Geometry: final body of the model. Coordinates: model frame, mm. A direction names the side the tool comes from. Coordinates: 2 decimals unless noted, no trailing zeros. Write each loop counter-clockwise with the first axis right and the second up, starting at its lowest first coordinate (ties: lowest second). Pieces come first, ordered by that corner, then holes. Notation, with made-up numbers: (69, -27) -> (91, -27) arc R21 ccw to (91, 12) -> close; hole circle Ø11 at (76.25, -1.5). An arc over 180 degrees is marked (long way). One line per item, written item: value.
Autodesk Inventor part; units mm, degrees
ref_plane "YZ Plane" through (0, 0, 0) normal (1, 0, 0) x (0, 1, 0)
ref_plane "XZ Plane" through (0, 0, 0) normal (0, 1, 0) x (-1, 0, 0)
ref_plane "XY Plane" through (0, 0, 0) normal (0, 0, 1) x (1, 0, 0)
sketch "Sketch1" plane through (0, 0, 0) normal (0, 0, 1) x (1, 0, 0)
  line L0 (35, -3.75) -> (-35, -3.75)
  line L1 (-35, -3.75) -> (-35, 3.75)
  line L2 (-35, 3.75) -> (35, 3.75)
  line L3 (35, 3.75) -> (35, -3.75)
  line L4 (35, -3.75) -> (-35, 3.75) construction
  line L5 (-35, -3.75) -> (35, 3.75) construction
  line L6 (21.5, -16.5) -> (-21.5, -16.5)
  line L7 (-21.5, -16.5) -> (-21.5, 16.5)
  line L8 (-21.5, 16.5) -> (21.5, 16.5)
  line L9 (21.5, 16.5) -> (21.5, -16.5)
  line L10 (21.5, -16.5) -> (-21.5, 16.5) construction
  line L11 (-21.5, -16.5) -> (21.5, 16.5) construction
  line L12 (-35, -3.75) -> (-21.5, -16.5)
  line L13 (-35, 3.75) -> (-21.5, 16.5)
  arc A0 (32.3113, 4.5234) -> (35, 3.75) centre (34.605, 7.4371) ccw
  line L14 (21.5, -16.5) -> (35, -3.75)
  line L15 (35, 3.75) -> (21.5, 16.5)
  point P0 (0, 0)
  dimension "d0" = 70
  dimension "d1" = 7.5
  dimension "d2" = 43
  dimension "d3" = 33
extrude "Extrusion1" add sketch "Sketch1" along normal blind 30
sketch "Sketch2" plane through (-21.5, -16.5, 0) normal (0, -1, 0) x (1, 0, 0)
  line L0 (43, 30) -> (0, 30)
  line L1 (43, 0) -> (0, 0)
  line L2 (0, 30) -> (43, 30)
  line L3 (43, 30) -> (43, 0)
  line L4 (43, 0) -> (0, 0)
  line L5 (0, 0) -> (0, 30)
  line L6 (21.5, 30) -> (24.75, 30)
  line L7 (56.5, 0) -> (56.5, 30)
  line L8 (56.5, 0) -> (56.5, 10)
  line L9 (24.75, 30) -> (29.6997, 25.0503)
  arc A0 (29.6997, 25.0503) -> (56.5, 10) centre (56.5, 41.387) ccw
  arc A1 (55.355, 10.0209) -> (56.5, 10) centre (56.5, 41.387) ccw
  line L10 (56.5, 10) -> (46.9475, 10)
  line L11 (21.5, 30) -> (21.5, 26.75)
  line L12 (21.5, 30) -> (18.25, 30)
  line L13 (-13.5, 0) -> (-13.5, 30)
  line L14 (18.25, 30) -> (13.3003, 25.0503)
  arc A2 (-13.5, 10) -> (13.3003, 25.0503) centre (-13.5, 41.387) ccw
  line L15 (43, 30) -> (56.5, 30)
  line L16 (43, 0) -> (43, 30)
  line L17 (56.5, 30) -> (43, 30)
  line L18 (43, 0) -> (43, 30)
  line L19 (56.5, 0) -> (43, 0)
  line L20 (56.5, 0) -> (56.5, 30)
  line L21 (43, 0) -> (56.5, 0)
  line L22 (43, 0) -> (56.5, 0)
  line L23 (56.5, 0) -> (56.5, 30)
  line L24 (43, 30) -> (56.5, 30)
  line L25 (43, 0) -> (43, 30)
  line L26 (56.5, 0) -> (56.5, 30)
  line L27 (56.5, 0) -> (56.5, 30)
  line L28 (56.5, 0) -> (43, 0)
  line L29 (43, 0) -> (43, 30)
  line L30 (56.5, 30) -> (43, 30)
  line L31 (56.5, 0) -> (56.5, 30)
  line L32 (43, 0) -> (56.5, 0)
  line L33 (0, 0) -> (43, 0)
  line L34 (-13.5, 0) -> (0, 0)
  line L35 (0, 0) -> (-13.5, 0)
  line L36 (43, 0) -> (0, 0)
  line L37 (56.5, 0) -> (43, 0)
  line L38 (43, 30) -> (56.5, 30)
  line L39 (56.5, 30) -> (43, 30)
  line L40 (43, 30) -> (0, 30)
  line L41 (0, 30) -> (-13.5, 30)
  line L42 (-13.5, 30) -> (0, 30)
  line L43 (0, 30) -> (43, 30)
  line L44 (0, 30) -> (43, 30)
  line L45 (0, 0) -> (43, 0)
  line L46 (43, 0) -> (0, 0)
  line L47 (0, 0) -> (0, 30)
  line L48 (43, 30) -> (0, 30)
  line L49 (43, 0) -> (43, 30)
  line L50 (0, 0) -> (43, 0)
  line L51 (43, 0) -> (43, 30)
  line L52 (0, 30) -> (43, 30)
  line L53 (0, 0) -> (0, 30)
  line L54 (0, 0) -> (0, 30)
  line L55 (0, 0) -> (0, 30)
  line L56 (0, 0) -> (-13.5, 0)
  line L57 (-13.5, 0) -> (-13.5, 30)
  line L58 (-13.5, 0) -> (-13.5, 30)
  line L59 (-13.5, 0) -> (0, 0)
  line L60 (0, 0) -> (-13.5, 0)
  line L61 (-13.5, 0) -> (-13.5, 30)
  line L62 (0, 30) -> (-13.5, 30)
  line L63 (0, 0) -> (0, 30)
  line L64 (-13.5, 0) -> (-13.5, 30)
  line L65 (-13.5, 0) -> (-13.5, 30)
  line L66 (-13.5, 0) -> (0, 0)
  line L67 (0, 0) -> (0, 30)
  line L68 (-13.5, 30) -> (0, 30)
  line L69 (-13.5, 0) -> (-13.5, 30)
  line L70 (-13.5, 30) -> (0, 30)
  line L71 (0, 30) -> (-13.5, 30)
  point P0 (21.5, 0)
  dimension "d6" = 3.25
  dimension "d7" = 10
  dimension "d8" = 7
  dimension "d9" = 45
extrude "Extrusion2" cut sketch "Sketch2" against normal blind 36.35 contours L3 A0 L9 L0 | L15 L7 A0 L3 | L14 A2 L5 L0 | L5 A2 L13 L41
sketch "Sketch3" plane through (0, 0, 0) normal (0, 0, -1) x (-1, 0, 0)
  line L0 (35, 3.75) -> (35, -3.75)
  circle A0 centre (29.3, 0) radius 3.1
  line L1 (32.4, 0) -> (24.3, 0)
  circle A1 centre (24.3, 0) radius 3.1
  line L2 (29.3, -3.1) -> (24.3, -3.1)
  line L3 (29.3, 3.1) -> (24.3, 3.1)
  line L4 (0, 0) -> (0, -2.435)
  circle A2 centre (-29.3, 0) radius 3.1
  line L5 (-32.4, 0) -> (-24.3, 0)
  circle A3 centre (-24.3, 0) radius 3.1
  line L6 (-29.3, -3.1) -> (-24.3, -3.1)
  line L7 (-29.3, 3.1) -> (-24.3, 3.1)
  dimension "d12" = 5.7
  dimension "d13" = 6.2
  dimension "d14" = 8.1
  dimension "d15" = 6.2
extrude "Extrusion3" cut sketch "Sketch3" against normal blind 36.35
properties part number "scanner"
(1) Section A-A (z = 2). Return the cut outline in (x, y).
Responses:
outline: (-35, -3.75) -> (-21.5, -16.5) -> (21.5, -16.5) -> (35, -3.75) -> (35, 3.75) -> (21.5, 16.5) -> (-21.5, 16.5) -> (-35, 3.75) -> close; hole (-29.3, -3.1) -> (-24.3, -3.1) arc R3.1 ccw to (-24.3, 3.1) -> (-29.3, 3.1) arc R3.1 ccw to start; hole (24.3, -3.1) -> (29.3, -3.1) arc R3.1 ccw to (29.3, 3.1) -> (24.3, 3.1) arc R3.1 ccw to start
(2) Pull-direction query (Y, two-part tool) for faces 1 (the flat face through (-28.34, -10.04, 4.98)), 2 (the flat face through (-35, 0, 5)), 3 (the flat face through (-27, 3.1, 6)); classes: released by +Y, released by -Y, zero draft, split by the parting line, or undercut.
Responses:
face 1: released by -Y
face 2: zero draft
face 3: undercut
(3) First-contact query: pin 1 (8 mm diameter, centred on y = 12.5, z = 4, fed in from -X); pin 2 (10 mm diameter, centred on x = -24.5, z = 9, fed in from -Y); pin 3 (6 mm diameter, centred on y = -1, z = 25.5, fed in from -X); pin 4 (3 mm diameter, centred on x = -10, y = -0.5, fed in from +Z). Flat tips, straight axial feed; report the tip coordinate or a pass-through.
Responses:
pin 1: stops at x = -29.97
pin 2: stops at y = -16.5
pin 3: stops at x = -9.93
pin 4: stops at z = 24.57
(4) Line query: line 1 (Z direction, x = -21.5, y = 6.5); line 2 (Y direction, x = -27, z = 6); line 3 (X direction, y = -2, z = 4.5). Output: solid intervals per line, ascending. Write a range as [from, to].
Responses:
line 1: z = [0, 13.05]
line 2: y = [-11.31, -3.1], [3.1, 11.31]
line 3: x = [-35, -31.67], [-21.93, 21.93], [31.67, 35]
(5) Section D-D (y = -10.5). Return the cut outline in (x, z).
Responses:
outline: (-27.85, 0) -> (27.85, 0) -> (27.85, 10.82) arc R31.39 cw to (8.2, 25.05) -> (3.25, 30) -> (-3.25, 30) -> (-8.2, 25.05) arc R31.39 cw to (-27.85, 10.82) -> close
(6) Section C-C (y = 0). Return the cut outline in (x, z), then the cut area to 3 significant figures.
Responses:
outline: (-35, 0) -> (-32.4, 0) -> (-32.4, 10.11) arc R31.39 cw to (-35, 10) -> close; (-21.2, 0) -> (21.2, 0) -> (21.2, 13.2) arc R31.39 cw to (8.2, 25.05) -> (3.25, 30) -> (-3.25, 30) -> (-8.2, 25.05) arc R31.39 cw to (-21.2, 13.2) -> close; (32.4, 0) -> (35, 0) -> (35, 10) arc R31.39 cw to (32.4, 10.11) -> close
area: 987 mm2
(7) Reachability of faces 4 (the flat face through (0, -16.5, 11)), 5 (the flat face through (27, 3.1, 6)) from +Z, -Z, +X, -X, +Y, -Y: full face, straight path, thin tool, end or side. Return the list, or none.
Responses:
face 4: +Z, -Z, +X, -X, -Y
face 5: +Z, -Z
(8) Section B-B (x = -26). Return the cut outline in (y, z).
Responses:
outline: (-12.25, 0) -> (-3.1, 0) -> (-3.1, 11.32) -> (-12.25, 11.32) -> close; (3.1, 0) -> (12.25, 0) -> (12.25, 11.32) -> (3.1, 11.32) -> close
